Here's how the part is built. I have some questions about the finished solid (model axes, mm). Coordinates: 2 decimals unless noted, no trailing zeros. Use a Markdown table: item, result.
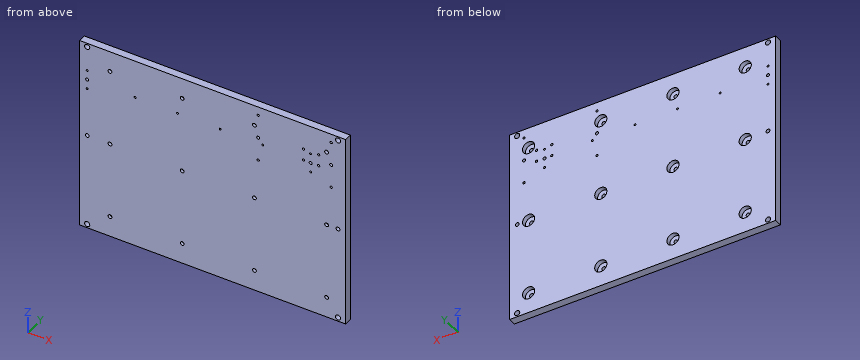
```python
from build123d import *

# Parameters (mm, degrees)
SKETCH2_W           = 920
SKETCH2_H           = 264
BOSS_EXTRUDE1_DEPTH = 10
SKETCH1_R           = 2.5
CUT_EXTRUDE2_DEPTH  = 18
SKETCH3_R           = 8
CUT_EXTRUDE3_DEPTH  = 6
SKETCH4_W           = 570
SKETCH4_H           = 264
CUT_EXTRUDE4_DEPTH  = 20
SKETCH7_R           = 3.4
SKETCH7_R_2         = 2.5
CUT_EXTRUDE5_DEPTH  = 20
SKETCH8_W           = 350
SKETCH8_H           = 5
CUT_EXTRUDE6_DEPTH  = 10
SKETCH9_R           = 1.25
SKETCH9_R_2         = 2
CUT_EXTRUDE7_DEPTH  = 10
SKETCH10_R          = 1.5
SKETCH10_R_2        = 2
CUT_EXTRUDE8_DEPTH  = 10


with BuildPart() as part:
    # Sketch2 → Boss-Extrude1 (new body)
    with BuildSketch(Plane(origin=(0, 0, 0), x_dir=(1, 0, 0), z_dir=(0, 1, 0))):
        with Locations((460, 132)):
            Rectangle(SKETCH2_W, SKETCH2_H)
    extrude(amount=BOSS_EXTRUDE1_DEPTH)

    # Sketch1 → Cut-Extrude2 (cut)
    with BuildSketch(Plane(origin=(0, 10, 0), x_dir=(1, 0, 0), z_dir=(0, 1, 0))):
        with Locations(Location((40, 32, 0), (0, 0, 270))):
            Circle(SKETCH1_R)
        with Locations(Location((135, 32, 0), (0, 0, 270))):
            Circle(SKETCH1_R)
        with Locations(Location((230, 32, 0), (0, 0, 270))):
            Circle(SKETCH1_R)
        with Locations(Location((325, 32, 0), (0, 0, 270))):
            Circle(SKETCH1_R)
        with Locations(Location((420, 32, 0), (0, 0, 270))):
            Circle(SKETCH1_R)
        with Locations(Location((515, 32, 0), (0, 0, 270))):
            Circle(SKETCH1_R)
        with Locations(Location((610, 32, 0), (0, 0, 270))):
            Circle(SKETCH1_R)
        with Locations(Location((705, 32, 0), (0, 0, 270))):
            Circle(SKETCH1_R)
        with Locations(Location((800, 32, 0), (0, 0, 270))):
            Circle(SKETCH1_R)
        with Locations(Location((895, 32, 0), (0, 0, 270))):
            Circle(SKETCH1_R)
        with Locations(Location((135, 132, 0), (0, 0, 270))):
            Circle(SKETCH1_R)
        with Locations(Location((230, 132, 0), (0, 0, 270))):
            Circle(SKETCH1_R)
        with Locations(Location((325, 132, 0), (0, 0, 270))):
            Circle(SKETCH1_R)
        with Locations(Location((420, 132, 0), (0, 0, 270))):
            Circle(SKETCH1_R)
        with Locations(Location((515, 132, 0), (0, 0, 270))):
            Circle(SKETCH1_R)
        with Locations(Location((610, 132, 0), (0, 0, 270))):
            Circle(SKETCH1_R)
        with Locations(Location((705, 132, 0), (0, 0, 270))):
            Circle(SKETCH1_R)
        with Locations(Location((800, 132, 0), (0, 0, 270))):
            Circle(SKETCH1_R)
        with Locations(Location((895, 132, 0), (0, 0, 270))):
            Circle(SKETCH1_R)
        with Locations(Location((135, 232, 0), (0, 0, 270))):
            Circle(SKETCH1_R)
        with Locations(Location((230, 232, 0), (0, 0, 270))):
            Circle(SKETCH1_R)
        with Locations(Location((325, 232, 0), (0, 0, 270))):
            Circle(SKETCH1_R)
        with Locations(Location((420, 232, 0), (0, 0, 270))):
            Circle(SKETCH1_R)
        with Locations(Location((515, 232, 0), (0, 0, 270))):
            Circle(SKETCH1_R)
        with Locations(Location((610, 232, 0), (0, 0, 270))):
            Circle(SKETCH1_R)
        with Locations(Location((705, 232, 0), (0, 0, 270))):
            Circle(SKETCH1_R)
        with Locations(Location((800, 232, 0), (0, 0, 270))):
            Circle(SKETCH1_R)
        with Locations(Location((895, 232, 0), (0, 0, 270))):
            Circle(SKETCH1_R)
        with Locations(Location((40, 132, 0), (0, 0, 270))):
            Circle(SKETCH1_R)
        with Locations(Location((40, 232, 0), (0, 0, 270))):
            Circle(SKETCH1_R)
    extrude(amount=-CUT_EXTRUDE2_DEPTH, mode=Mode.SUBTRACT)

    # Sketch3 → Cut-Extrude3 (cut)
    with BuildSketch(Plane(origin=(0, 10, 0), x_dir=(1, 0, 0), z_dir=(0, 1, 0))):
        with Locations(Location((40, 32, 0), (0, 0, 270))):
            Circle(SKETCH3_R)
        with Locations(Location((135, 32, 0), (0, 0, 270))):
            Circle(SKETCH3_R)
        with Locations(Location((230, 32, 0), (0, 0, 270))):
            Circle(SKETCH3_R)
        with Locations(Location((325, 32, 0), (0, 0, 270))):
            Circle(SKETCH3_R)
        with Locations(Location((420, 32, 0), (0, 0, 270))):
            Circle(SKETCH3_R)
        with Locations(Location((515, 32, 0), (0, 0, 270))):
            Circle(SKETCH3_R)
        with Locations(Location((610, 32, 0), (0, 0, 270))):
            Circle(SKETCH3_R)
        with Locations(Location((705, 32, 0), (0, 0, 270))):
            Circle(SKETCH3_R)
        with Locations(Location((800, 32, 0), (0, 0, 270))):
            Circle(SKETCH3_R)
        with Locations(Location((895, 32, 0), (0, 0, 270))):
            Circle(SKETCH3_R)
        with Locations(Location((135, 132, 0), (0, 0, 270))):
            Circle(SKETCH3_R)
        with Locations(Location((230, 132, 0), (0, 0, 270))):
            Circle(SKETCH3_R)
        with Locations(Location((325, 132, 0), (0, 0, 270))):
            Circle(SKETCH3_R)
        with Locations(Location((420, 132, 0), (0, 0, 270))):
            Circle(SKETCH3_R)
        with Locations(Location((515, 132, 0), (0, 0, 270))):
            Circle(SKETCH3_R)
        with Locations(Location((610, 132, 0), (0, 0, 270))):
            Circle(SKETCH3_R)
        with Locations(Location((705, 132, 0), (0, 0, 270))):
            Circle(SKETCH3_R)
        with Locations(Location((800, 132, 0), (0, 0, 270))):
            Circle(SKETCH3_R)
        with Locations(Location((895, 132, 0), (0, 0, 270))):
            Circle(SKETCH3_R)
        with Locations(Location((135, 232, 0), (0, 0, 270))):
            Circle(SKETCH3_R)
        with Locations(Location((230, 232, 0), (0, 0, 270))):
            Circle(SKETCH3_R)
        with Locations(Location((325, 232, 0), (0, 0, 270))):
            Circle(SKETCH3_R)
        with Locations(Location((420, 232, 0), (0, 0, 270))):
            Circle(SKETCH3_R)
        with Locations(Location((515, 232, 0), (0, 0, 270))):
            Circle(SKETCH3_R)
        with Locations(Location((610, 232, 0), (0, 0, 270))):
            Circle(SKETCH3_R)
        with Locations(Location((705, 232, 0), (0, 0, 270))):
            Circle(SKETCH3_R)
        with Locations(Location((800, 232, 0), (0, 0, 270))):
            Circle(SKETCH3_R)
        with Locations(Location((895, 232, 0), (0, 0, 270))):
            Circle(SKETCH3_R)
        with Locations(Location((40, 132, 0), (0, 0, 270))):
            Circle(SKETCH3_R)
        with Locations(Location((40, 232, 0), (0, 0, 270))):
            Circle(SKETCH3_R)
    extrude(amount=-CUT_EXTRUDE3_DEPTH, mode=Mode.SUBTRACT)

    # Sketch4 → Cut-Extrude4 (cut)
    with BuildSketch(Plane(origin=(0, 10, 0), x_dir=(1, 0, 0), z_dir=(0, 1, 0))):
        with Locations((635, 132)):
            Rectangle(SKETCH4_W, SKETCH4_H)
    extrude(amount=-CUT_EXTRUDE4_DEPTH, mode=Mode.SUBTRACT)

    # Sketch7 → Cut-Extrude5 (cut)
    with BuildSketch(Plane(origin=(0, 10, 0), x_dir=(1, 0, 0), z_dir=(0, 1, 0))):
        with Locations(Location((10, 254, 0), (0, 0, 270))):
            Circle(SKETCH7_R)
        with Locations(Location((340, 254, 0), (0, 0, 270))):
            Circle(SKETCH7_R)
        with Locations(Location((340, 10, 0), (0, 0, 270))):
            Circle(SKETCH7_R)
        with Locations(Location((10, 10, 0), (0, 0, 270))):
            Circle(SKETCH7_R)
        with Locations(Location((10, 132, 0), (0, 0, 270))):
            Circle(SKETCH7_R_2)
        with Locations(Location((340, 132, 0), (0, 0, 270))):
            Circle(SKETCH7_R_2)
    extrude(amount=-CUT_EXTRUDE5_DEPTH, mode=Mode.SUBTRACT)

    # Sketch8 → Cut-Extrude6 (cut)
    with BuildSketch(Plane(origin=(0, 10, 0), x_dir=(1, 0, 0), z_dir=(0, 1, 0))):
        with Locations((175, 261.5)):
            Rectangle(SKETCH8_W, SKETCH8_H)
        with Locations((175, 2.5)):
            Rectangle(SKETCH8_W, SKETCH8_H)
    extrude(amount=-CUT_EXTRUDE6_DEPTH, mode=Mode.SUBTRACT)

    # Sketch9 → Cut-Extrude7 (cut)
    with BuildSketch(Plane(origin=(0, 10, 0), x_dir=(1, 0, 0), z_dir=(0, 1, 0))):
        with Locations(Location((10, 67.5, 0), (0, 0, 270))):
            Circle(SKETCH9_R)
        with Locations(Location((10, 42.5, 0), (0, 0, 270))):
            Circle(SKETCH9_R)
        with Locations(Location((304, 67.5, 0), (0, 0, 90))):
            Circle(SKETCH9_R)
        with Locations(Location((304, 42.5, 0), (0, 0, 90))):
            Circle(SKETCH9_R)
        with Locations(Location((73, 55, 0), (0, 0, 270))):
            Circle(SKETCH9_R)
        with Locations(Location((129, 55, 0), (0, 0, 270))):
            Circle(SKETCH9_R)
        with Locations(Location((185, 55, 0), (0, 0, 90))):
            Circle(SKETCH9_R)
        with Locations(Location((241, 55, 0), (0, 0, 90))):
            Circle(SKETCH9_R)
        with Locations(Location((10, 55, 0), (0, 0, 270))):
            Circle(SKETCH9_R_2)
        with Locations(Location((304, 55, 0), (0, 0, 90))):
            Circle(SKETCH9_R_2)
    extrude(amount=-CUT_EXTRUDE7_DEPTH, mode=Mode.SUBTRACT)

    # Sketch10 → Cut-Extrude8 (cut)
    with BuildSketch(Plane(origin=(0, 10, 0), x_dir=(1, 0, 0), z_dir=(0, 1, 0))):
        with Locations(Location((235, 78.013636364, 0), (0, 0, 270))):
            Circle(SKETCH10_R)
        with Locations(Location((235, 16.486363636, 0), (0, 0, 270))):
            Circle(SKETCH10_R)
        with Locations(Location((294.500010803, 39.75, 0), (0, 0, 270))):
            Circle(SKETCH10_R)
        with Locations(Location((314.500010803, 54.75, 0), (0, 0, 270))):
            Circle(SKETCH10_R)
        with Locations(Location((331, 16.486363636, 0), (0, 0, 270))):
            Circle(SKETCH10_R)
        with Locations(Location((331, 47.25, 0), (0, 0, 270))):
            Circle(SKETCH10_R_2)
        with Locations(Location((331, 78.013636364, 0), (0, 0, 270))):
            Circle(SKETCH10_R)
        with Locations(Location((235, 47.25, 0), (0, 0, 270))):
            Circle(SKETCH10_R_2)
        with Locations(Location((294.500010803, 54.75, 0), (0, 0, 270))):
            Circle(SKETCH10_R)
        with Locations(Location((314.500010803, 39.75, 0), (0, 0, 270))):
            Circle(SKETCH10_R)
    extrude(amount=-CUT_EXTRUDE8_DEPTH, mode=Mode.SUBTRACT)


solid = part.part
```
Q1. I want a section at A-A, the plane y = 6.75. Give the number of separate pieces and of enclosed holes in the cut face, then the cut area to 3 significant figures.
Check values:
| item | result |
|---|---|
| separate pieces | 1 |
| enclosed holes | 38 |
| area | 86,200 mm^2 |
Q2. Will this pin go through, and if not, where does the flat tip stop? P1, Ø5, axis at x = 38, z = -30.5, coming from the +Y side.
Check values:
| item | result |
|---|---|
| P1 | y = 4 |
Q3. Please list where these lines run through material, in increasing order: L1, parallel to Z at x = 325, y = 1.2; L2, parallel to X at y = 7.5, z = -67.5; L3, parallel to X at y = 8, z = -29. Write a range as from..to.
Check values:
| item | result |
|---|---|
| L1 | -259..-234.5, -229.5..-134.5, -129.5..-34.5, -29.5..-5 |
| L2 | 0..8.75, 11.25..302.75, 305.25..350 |
| L3 | 0..32.58, 47.42..127.58, 142.42..222.58, 237.42..317.58, 332.42..350 |
